Model file for the job. Use its own axes, mm. A direction names the side the tool comes from. Give positions to 0.01 mm unless a question says otherwise; leave off trailing zeros. Loops run counter-clockwise (first coordinate to the right, second up) from the corner with the lowest first, then second, coordinate; pieces in that order, holes last. Notation, with made-up numbers: (39, 17) - (51, 17) arc R25 ccw to (51, 38) - close; hole circle Ø4 at (18.25, -8.5). An arc over 180 degrees is marked (long way). Use a Markdown table: item, result.
from build123d import *

# Parameters (mm, degrees)
SKETCH1_R                = 14
SKETCH1_R_2              = 4.1
BOSS_EXTRUDE1_DEPTH      = 2.5
SKETCH2_R                = 5
SKETCH2_R_2              = 4.1
BOSS_EXTRUDE2_DEPTH      = 2.5
M2_5X0_45_TAPPED_HOLE1_D = 2.05
SKETCH7_R                = 5
CUT_EXTRUDE1_DEPTH       = 1.5


with BuildPart() as part:
    # Sketch1 → Boss-Extrude1 (new body)
    with BuildSketch(Plane(origin=(0, 0, 0), x_dir=(0, 0, -1), z_dir=(1, 0, 0))):
        Circle(SKETCH1_R)
        Circle(SKETCH1_R_2, mode=Mode.SUBTRACT)
    extrude(amount=BOSS_EXTRUDE1_DEPTH)

    # Sketch2 → Boss-Extrude2 (add)
    with BuildSketch(Plane(origin=(2.5, 0, 0), x_dir=(0, 0, -1), z_dir=(1, 0, 0))):
        Circle(SKETCH2_R)
        Circle(SKETCH2_R_2, mode=Mode.SUBTRACT)
    extrude(amount=BOSS_EXTRUDE2_DEPTH)

    # M2.5x0.45 Tapped Hole1 (through all)
    with Locations(Plane(origin=(5, 0, 0), x_dir=(0, 0, -1), z_dir=(1, 0, 0))):
        with Locations((0, 11), (7.778174593, 7.778174593), (11, 0), (7.778174593, -7.778174593), (0, -11), (-7.778174593, -7.778174593), (-11, 0), (-7.778174593, 7.778174593), (0, 0)):
            Hole(M2_5X0_45_TAPPED_HOLE1_D / 2)

    # Sketch7 → Cut-Extrude1 (cut)
    with BuildSketch(Plane.ZY):
        Circle(SKETCH7_R)
    extrude(amount=-CUT_EXTRUDE1_DEPTH, mode=Mode.SUBTRACT)


solid = part.part
(1) Slice it at B-B, the plane z = -0.25. Write the cut outline in (x, y).
Computed:
| item | result |
|---|---|
| outline | (0, -14) - (2.5, -14) - (2.5, -11.99) - (0, -11.99) - close; (0, -10.01) - (2.5, -10.01) - (2.5, -4.99) - (5, -4.99) - (5, -4.09) - (1.5, -4.09) - (1.5, -4.99) - (0, -4.99) - close; (0, 4.99) - (1.5, 4.99) - (1.5, 4.09) - (5, 4.09) - (5, 4.99) - (2.5, 4.99) - (2.5, 10.01) - (0, 10.01) - close; (0, 11.99) - (2.5, 11.99) - (2.5, 14) - (0, 14) - close |
(2) Slice it at C-C, the plane z = -3.5. Write the cut outline in (x, y), plus the area to 3 significant figures.
Computed:
| item | result |
|---|---|
| outline | (0, -13.56) - (2.5, -13.56) - (2.5, -3.57) - (5, -3.57) - (5, -2.14) - (1.5, -2.14) - (1.5, -3.57) - (0, -3.57) - close; (0, 3.57) - (1.5, 3.57) - (1.5, 2.14) - (5, 2.14) - (5, 3.57) - (2.5, 3.57) - (2.5, 13.56) - (0, 13.56) - close |
| area | 60.0 mm² |
(3) Slice it at D-D, the plane y = -3.25. Write the cut outline in (x, z), plus the area to 3 significant figures.
Computed:
| item | result |
|---|---|
| outline | (0, -13.62) - (2.5, -13.62) - (2.5, -3.8) - (5, -3.8) - (5, -2.5) - (1.5, -2.5) - (1.5, -3.8) - (0, -3.8) - close; (0, 3.8) - (1.5, 3.8) - (1.5, 2.5) - (5, 2.5) - (5, 3.8) - (2.5, 3.8) - (2.5, 13.62) - (0, 13.62) - close |
| area | 58.2 mm² |
(4) Slice it at A-A, the plane y = 0. Write the cut outline in (x, z) (3 decimals), plus the area to 4 significant figures.
Computed:
| item | result |
|---|---|
| outline | (0, -14) - (2.5, -14) - (2.5, -12.025) - (0, -12.025) - close; (0, -9.975) - (2.5, -9.975) - (2.5, -5) - (5, -5) - (5, -4.1) - (1.5, -4.1) - (1.5, -5) - (0, -5) - close; (0, 5) - (1.5, 5) - (1.5, 4.1) - (5, 4.1) - (5, 5) - (2.5, 5) - (2.5, 9.975) - (0, 9.975) - close; (0, 12.025) - (2.5, 12.025) - (2.5, 14) - (0, 14) - close |
| area | 41.05 mm² |
(5) 3-axis set-ups, long thin cutter, end or side, ignore diameter. For faces 1 (the cylindrical face through (1.23, -6.76, -7.91)), 2 (the flat face through (2.5, -6, 0)), 3 (the flat face through (1.5, 2, -4)): which of +Z, -Z, +X, -X, +Y, -Y reach the whole face in a straight line?
Computed:
| item | result |
|---|---|
| face 1 | +X, -X |
| face 2 | +X |
| face 3 | -X |
(6) Pin check, flat tips, straight feed: P1, Ø6, axis at y = -10.5, z = -8, coming from the +X side; P2, Ø1.8, axis at y = 7.78, z = -7.78, coming from the -X side; P3, Ø3, axis at x = 4.5, z = -2, coming from the +Y side. Stop position of each tip, or through.
Computed:
| item | result |
|---|---|
| P1 | x = 2.5 |
| P2 | through |
| P3 | y = 4.97 |
(7) Drill centre lines: probe 1 along X at (y, z) = (-6, 6.75); probe 2 along Y at (x, z) = (1.7, -3.5); probe 3 along Z at (x, y) = (4.45, 1). Where is each one in solid material? Low to high. Write a range as [from, to].
Computed:
| item | result |
|---|---|
| probe 1 | [0, 2.5] |
| probe 2 | [-13.56, -2.14], [2.14, 13.56] |
| probe 3 | [-4.9, -3.98], [3.98, 4.9] |
(8) Mould opens along Z. For faces 4 (the cylindrical face through (0.74, -4.88, -1.08)), 5 (the flat face through (0, -6, 0)), 6 (the cylindrical face through (1.232, -5.362, -12.932)) say: pulls with the +Z half, pulls with the -Z half, needs draft (parallel to the pull), parting line crosses it, or undercut.
Computed:
| item | result |
|---|---|
| face 4 | undercut |
| face 5 | needs draft |
| face 6 | parting line crosses it |
